from build123d import *

# Parameters (mm, degrees)
BASPROSKE_W        = 16
BASPROSKE_H        = 11
SKETCH1_R          = 1
CUT_EXTRUDE1_DEPTH = 30
TOOTHCUT_DEPTH     = 23.315913604
TEETHCUTS_COUNT    = 20
TEETHCUTS_ANGLE    = 342
BORSKE_R           = 3
BORE_DEPTH         = 50.0000508


with BuildPart() as part:
    # BasProSke → Base-Revolve (revolve)
    with BuildSketch(Plane(origin=(0, 0, 0), x_dir=(1, 0, 0), z_dir=(0, 1, 0)), mode=Mode.PRIVATE) as base_revolve_sk:
        with Locations((8, 5.5)):
            Rectangle(BASPROSKE_W, BASPROSKE_H)
    revolve(base_revolve_sk.sketch.rotate(Axis((-10, 0, 0), (1, 0, 0)), 180), axis=Axis((-10, 0, 0), (1, 0, 0)))

    # Sketch1 → Cut-Extrude1 (cut)
    with BuildSketch(Plane(origin=(16, 0, 0), x_dir=(0, 0, -1), z_dir=(1, 0, 0))):
        with Locations((3.5, 3.5)):
            Circle(SKETCH1_R)
        with Locations((-3.5, 3.5)):
            Circle(SKETCH1_R)
        with Locations((-3.5, -3.5)):
            Circle(SKETCH1_R)
        with Locations((3.5, -3.5)):
            Circle(SKETCH1_R)
    extrude(amount=-CUT_EXTRUDE1_DEPTH, mode=Mode.SUBTRACT)

    # TooCutSke → ToothCut (cut, through all)
    with BuildSketch(Plane(origin=(0, 0, 0), x_dir=(0, 0, -1), z_dir=(1, 0, 0))):
        with BuildLine():
            ThreePointArc((0.499924007, 8.734705318), (0, 8.749), (-0.499924007, 8.734705318))
            ThreePointArc((-0.499924007, 8.734705318), (-0.824302243, 9.905497836), (-1.485192705, 10.924909509))
            ThreePointArc((-1.485192705, 10.924909509), (0, 11.0254), (1.485192705, 10.924909509))
            ThreePointArc((1.485192705, 10.924909509), (0.824302243, 9.905497836), (0.499924007, 8.734705318))
        make_face()
    toothcut = extrude(amount=TOOTHCUT_DEPTH, mode=Mode.SUBTRACT)

    # TeethCuts: ToothCut ×20 about axis
    teethcuts_axis = Axis((-10, 0, 0), (1, 0, 0))
    for i in range(1, TEETHCUTS_COUNT):
        add(toothcut.rotate(teethcuts_axis, i * TEETHCUTS_ANGLE / (TEETHCUTS_COUNT - 1)), mode=Mode.SUBTRACT)

    # BorSke → Bore (cut, symmetric)
    with BuildSketch(Plane(origin=(0, 0, 0), x_dir=(0, 0, -1), z_dir=(1, 0, 0))):
        with Locations(Location((0, 0, 0), (0, 0, 180))):
            Circle(BORSKE_R)
    extrude(amount=BORE_DEPTH, both=True, mode=Mode.SUBTRACT)


solid = part.part
Input: part model. Units: mm. Frame: model coordinates. A direction names the side the tool comes from. Round coordinates to 2 decimals unless told otherwise and drop trailing zeros. Order: outer loops, then holes, each group sorted by start corner. A loop starts at its lowest first (then second) coordinate and runs counter-clockwise, first axis right, second up. Notation, with made-up numbers: (-13.75, 71) - (40.25, 71) arc R10 ccw to (40.25, 82) - close; hole circle Ø1 at (41, -10.5). An arc over 180 degrees is marked (long way). Answer as a JSON object with one key per item and string values. Group by question number.
(1) Cut plane D-D (x = 2). Count the separate pieces of the cut face and the enclosed holes in it, then the cut area to 3 significant figures.
(2) Reachability of faces 1 (the face through (7.89, 3.85, 9.17)), 2 (the face through (7.89, 9.64, -2.28)), 3 (the face through (7.888, 0.811, -9.876)), 4 (the face through (7.888, 9.907, -0.825)), 5 (the face through (7.89, -7.53, 6.49)) from +Z, -Z, +X, -X, +Y, -Y: full face, straight path, thin tool, end or side. Return the list, or none.
(3) Cut plane B-B (z = 3.5). Return loops of the section in (x, y), then the cut area to 3 significant figures.
(4) Material intervals for probe 1 along Y at (x, z) = (7.25, 3.5); probe 2 along Y at (x, z) = (9, 8.5); probe 3 along Y at (x, z) = (15.25, 0), sorted ascending. Write a range as from..to.
(5) Cut plane A-A (y = 0). Return loops of the section in (x, z), then the cut area to 3 significant figures.
(6) Pin query (flat end, axial travel): P1, Ø3, axis at x = 3.5, y = -3, coming from the +Z side; P2, Ø8, axis at x = 3, y = 8.5, coming from the -Z side; P3, Ø3, axis at x = 4, z = -5, coming from the -Y side. Return the tip coordinate at first contact, or that it passes through.
Here are the results:
{
 "1": {"separate pieces": "1", "enclosed holes": "5", "area": "262 mm^2"},
 "2": {"face 1": "+Z, +X, -X", "face 2": "+X, -X", "face 3": "-Z, +X, -X", "face 4": "+X, -X, +Y", "face 5": "+X, -X, -Y"},
 "3": {"outline": "(0, -8.73) - (16, -8.73) - (16, -4.5) - (0, -4.5) - close; (0, -2.5) - (16, -2.5) - (16, 2.5) - (0, 2.5) - close; (0, 4.5) - (16, 4.5) - (16, 8.73) - (0, 8.73) - close", "area": "215 mm^2"},
 "4": {"probe 1": "y = -8.73..-4.5, -2.5..2.5, 4.5..8.73", "probe 2": "y = -5.16..-3.36, -2.23..2.23, 3.36..5.16", "probe 3": "y = -8.75..-3, 3..8.75"},
 "5": {"outline": "(0, -8.75) - (16, -8.75) - (16, -3) - (0, -3) - close; (0, 3) - (16, 3) - (16, 8.75) - (0, 8.75) - close", "area": "184 mm^2"},
 "6": {"P1": "stops at z = 10.9", "P2": "stops at z = -9.92", "P3": "stops at y = -9.92"}
}
